from build123d import *

# Parameters (mm, degrees)
SKETCH1_R           = 3.175
BOSS_EXTRUDE1_DEPTH = 3.175
CUT_EXTRUDE1_DEPTH  = 85.471


with BuildPart() as part:
    # Sketch1 → Boss-Extrude1 (new body)
    with BuildSketch(Plane.XY):
        with BuildLine():
            Line((3.175, 0), (34.925, 0))
            ThreePointArc((34.925, 0), (37.17006403, 0.92993597), (38.1, 3.175))
            Line((38.1, 3.175), (38.1, 98.425))
            ThreePointArc((38.1, 98.425), (37.17006403, 100.67006403), (34.925, 101.6))
            Line((34.925, 101.6), (3.175, 101.6))
            ThreePointArc((3.175, 101.6), (0.92993597, 100.67006403), (0, 98.425))
            Line((0, 98.425), (0, 3.175))
            ThreePointArc((0, 3.175), (0.92993597, 0.92993597), (3.175, 0))
        make_face()
        with Locations((19.05, 50.8)):
            Circle(SKETCH1_R, mode=Mode.SUBTRACT)
        with Locations((19.05, 76.2)):
            Circle(SKETCH1_R, mode=Mode.SUBTRACT)
        with BuildLine():
            Line((6.35, 6.35), (31.75, 6.35))
            ThreePointArc((31.75, 6.35), (32.872532015, 6.814967985), (33.3375, 7.9375))
            Line((33.3375, 7.9375), (33.3375, 33.3375))
            ThreePointArc((33.3375, 33.3375), (32.872532015, 34.460032015), (31.75, 34.925))
            Line((31.75, 34.925), (6.35, 34.925))
            ThreePointArc((6.35, 34.925), (5.227467985, 34.460032015), (4.7625, 33.3375))
            Line((4.7625, 33.3375), (4.7625, 7.9375))
            ThreePointArc((4.7625, 7.9375), (5.227467985, 6.814967985), (6.35, 6.35))
        make_face(mode=Mode.SUBTRACT)
    extrude(amount=BOSS_EXTRUDE1_DEPTH)

    # Sketch2 → Cut-Extrude1 (cut)
    with BuildSketch(Plane.ZY):
        Polygon((0.79375, 0), (3.175, 2.38125), (3.175, 0), align=None)
    extrude(amount=-CUT_EXTRUDE1_DEPTH, mode=Mode.SUBTRACT)


solid = part.part
Model file for the job. Use its own axes, mm. A direction names the side the tool comes from. Give positions to 0.01 mm unless a question says otherwise; leave off trailing zeros. Order: outer loops, then holes, each group sorted by start corner. A loop starts at its lowest first (then second) coordinate and runs counter-clockwise, first axis right, second up. Notation, with made-up numbers: (-17.75, -40) -> (8.25, -40) arc R22 ccw to (8.25, -11) -> close; hole circle Ø8 at (-8, 48.5). An arc over 180 degrees is marked (long way). Use CSV: the item, a comma, the result in double quotes.
1. Band-saw the part on D-D, the plane x = 19.05. Give the cut face in (y, z) (3 decimals).
Outcome:
outline,"(0, 0) -> (6.35, 0) -> (6.35, 3.175) -> (2.381, 3.175) -> (0, 0.794) -> close; (34.925, 0) -> (47.625, 0) -> (47.625, 3.175) -> (34.925, 3.175) -> close; (53.975, 0) -> (73.025, 0) -> (73.025, 3.175) -> (53.975, 3.175) -> close; (79.375, 0) -> (101.6, 0) -> (101.6, 3.175) -> (79.375, 3.175) -> close"
2. Drill centre lines: line 1 along Y through (x, z) = (19.05, 1.6) (3 decimals); line 2 along Y through (x, z) = (29.5, 0.9) (3 decimals); line 3 along X through (y, z) = (8.5, 0.25). Where is each one in solid material? Low to high. Write a range as from..to.
Outcome:
line 1,"0.806..6.35, 34.925..47.625, 53.975..73.025, 79.375..101.6"
line 2,"0.106..6.35, 34.925..101.6"
line 3,"0..4.76, 33.34..38.1"
3. Mould opens along X. For faces 3 (the cylindrical face through (37.51, 1.33, 1.21)), 4 (the flat face through (33.338, 20, 2)), 5 (the flat face through (19, 64, 3.175)) say: +X half, -X half, draft (parallel to the pull), parting line (faces both ways), or undercut.
Outcome:
face 3,"+X half"
face 4,"undercut"
face 5,"draft"
4. Band-saw the part on B-B, the plane x = 30.5. Give the cut face in (y, z) (3 decimals), then the cut area to 3 significant figures.
Outcome:
outline,"(0, 0) -> (6.35, 0) -> (6.35, 3.175) -> (2.381, 3.175) -> (0, 0.794) -> close; (34.925, 0) -> (101.6, 0) -> (101.6, 3.175) -> (34.925, 3.175) -> close"
area,"229 mm²"
5. Band-saw the part on C-C, the plane z = 1.9. Count the separate pieces of the cut face and the enclosed holes in it, then the cut area to 3 significant figures.
Outcome:
separate pieces,"1"
enclosed holes,"3"
area,"2,950 mm²"
6. Drop a flat-ended pin along its axis: pin 1 (1 mm diameter, centred on x = 18.5, z = 2, fed in from -Y). Give the stop position or say it passes through.
Outcome:
pin 1,"y = 0.71"
7. Band-saw the part on A-A, the plane y = 15.5. Give the cut face in (x, z) (1 decimal), then the cut area to 3 significant figures.
Outcome:
outline,"(0, 0) -> (4.8, 0) -> (4.8, 3.2) -> (0, 3.2) -> close; (33.3, 0) -> (38.1, 0) -> (38.1, 3.2) -> (33.3, 3.2) -> close"
area,"30.2 mm²"
8. 3-axis set-ups, long thin cutter, end or side, ignore diameter. For faces 1 (the flat face through (19, 34.925, 2)), 2 (the cylindrical face through (0.554, 1.383, 1.212)): which of +Z, -Z, +X, -X, +Y, -Y reach the whole face in a straight line?
Outcome:
face 1,"+Z, -Z"
face 2,"+Z, -Z, -X, -Y"
